from build123d import *

# Parameters (mm, degrees)
SKETCH1_R            = 6.096
BOSS_EXTRUDE8_DEPTH  = 40.767
SKETCH7_R            = 1.143
BOSS_EXTRUDE10_DEPTH = 3.3782
SKETCH8_R            = 1.143
BOSS_EXTRUDE12_DEPTH = 3.3782


with BuildPart() as part:
    # Sketch1 → Boss-Extrude8 (new body)
    with BuildSketch(Plane(origin=(0, 0, 0), x_dir=(1, 0, 0), z_dir=(0, 1, 0))):
        Circle(SKETCH1_R)
    extrude(amount=BOSS_EXTRUDE8_DEPTH)

    # Sketch7 → Boss-Extrude10 (add)
    with BuildSketch(Plane.XZ):
        Circle(SKETCH7_R)
    extrude(amount=BOSS_EXTRUDE10_DEPTH)

    # Sketch8 → Boss-Extrude12 (add)
    with BuildSketch(Plane(origin=(0, 40.767, 0), x_dir=(1, 0, 0), z_dir=(0, 1, 0))):
        Circle(SKETCH8_R)
    extrude(amount=BOSS_EXTRUDE12_DEPTH)


solid = part.part
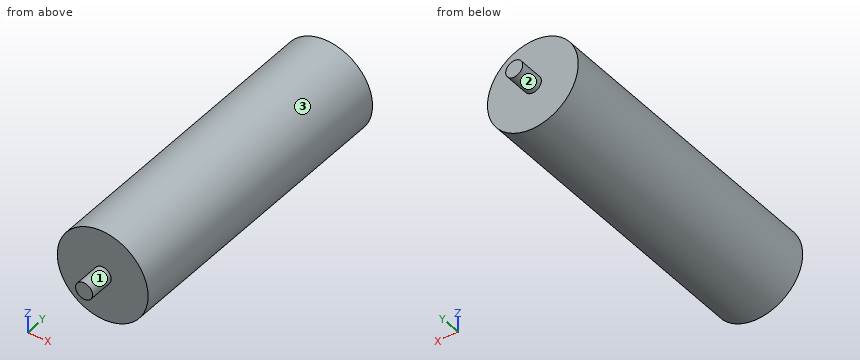
Can you work these out from the model? Positions are in its coordinate system, mm. Face numbers are marked on the shaded views. A direction names the side the tool comes from. Round coordinates to 2 decimals unless told otherwise and drop trailing zeros. Loops run counter-clockwise (first coordinate to the right, second up) from the corner with the lowest first, then second, coordinate; pieces in that order, holes last. Notation, with made-up numbers: (-18, 73.25) - (40, 73.25) arc R21 ccw to (40, 97.25) - close; hole circle Ø1 at (29.25, 74.25). An arc over 180 degrees is marked (long way). Answer in a Markdown table with one row per item. Add a question column.
Q1. I want a section at C-C on y = 3. List the corners of the cut face in (x, z) for me.
Q2. Which directions (+Z, -Z, +X, -X, +Y, -Y) give clear straight access to the entire face, cutting with the end or side of a thin tool? Please do the marked faces 1, 2 and 3.
Q3. I need wall thicknesses on L1, parallel to Y at x = -4.5, z = -2.75; L2, parallel to X at y = 2.5, z = 4; L3, parallel to X at y = 22, z = -3.5. Which ranges of each line are inside material? Lowest first, please.
Q4. I want a section at B-B on z = 0. List the corners of the cut face in (x, y) for me.
Q5. I want a section at D-D on z = -4.5. List the corners of the cut face in (x, y) for me.
Q6. I want a section at A-A on x = 0. List the corners of the cut face in (y, z) for me, and give its area (3 significant figures).
Q7. For pin 1 Ø3 at (x, y) = (-2.5, 26.5) entering from -Z; pin 2 Ø4 at (x, z) = (-1.5, -4) entering from +Y; pin 3 Ø1 at (x, y) = (-4, 16.5) entering from -Z; pin 4 Ø4 at (x, y) = (1, 10) entering from -Z, each with a flat end and sliding along its axis, tell me the tip position at first contact or that it passes through.
A:
| question | item | result |
|---|---|---|
| 1 | outline | circle Ø12.19 at (0, 0) |
| 2 | face 1 | -Y |
| 2 | face 2 | +Y |
| 2 | face 3 | +Y, -Y |
| 3 | L1 | 0 to 40.77 |
| 3 | L2 | -4.6 to 4.6 |
| 3 | L3 | -4.99 to 4.99 |
| 4 | outline | (-6.1, 0) - (-1.14, 0) - (-1.14, -3.38) - (1.14, -3.38) - (1.14, 0) - (6.1, 0) - (6.1, 40.77) - (1.14, 40.77) - (1.14, 44.15) - (-1.14, 44.15) - (-1.14, 40.77) - (-6.1, 40.77) - close |
| 5 | outline | (-4.11, 0) - (4.11, 0) - (4.11, 40.77) - (-4.11, 40.77) - close |
| 6 | outline | (-3.38, -1.14) - (0, -1.14) - (0, -6.1) - (40.77, -6.1) - (40.77, -1.14) - (44.15, -1.14) - (44.15, 1.14) - (40.77, 1.14) - (40.77, 6.1) - (0, 6.1) - (0, 1.14) - (-3.38, 1.14) - close |
| 6 | area | 512 mm^2 |
| 7 | pin 1 | z = -6.01 |
| 7 | pin 2 | y = 40.77 |
| 7 | pin 3 | z = -4.99 |
| 7 | pin 4 | z = -6.1 |
